Source: CAD feature listing. Evaluate the final solid. Frame: model axes, mm. Face numbers are marked on the shaded views. A direction names the side the tool comes from. Round coordinates to 2 decimals unless told otherwise and drop trailing zeros. Order: outer loops, then holes, each group sorted by start corner. A loop starts at its lowest first (then second) coordinate and runs counter-clockwise, first axis right, second up. Notation, with made-up numbers: (48, -7) -> (65, -7) arc R17 cw to (65, 11) -> close; hole circle Ø7 at (37, -23.75). An arc over 180 degrees is marked (long way). Write item = value, one per line. Start each with the question number.
(1) Cut plane B-B on y = 38. Return the cut outline in (x, z).
(2) Ray query, line 1 (Y direction, x = 43.5, z = 45.5); line 2 (Z direction, x = 41.5, y = -24); line 3 (Z direction, x = -2.5, y = -39). Return the intervals inside material, ascending.
(3) Cut plane A-A on x = -25.5. Return the cut outline in (y, z).
(4) Cut plane C-C on z = 36. Return the cut outline in (x, y), then the cut area to 3 significant figures.
(5) Contact query for flat-ended pins moving along their axis: pin 1 Ø6 at (x, y) = (-11, -40.5) entering from +Z; pin 2 Ø9 at (x, y) = (12, -28) entering from +Z; pin 3 Ø2.5 at (x, z) = (15, 53.5) entering from +Y. Output: stop coordinate, or through.
(6) Reachability of the marked faces 1, 2 and 3 from +Z, -Z, +X, -X, +Y, -Y: full face, straight path, thin tool, end or side. Return the list, or none.
from build123d import *

# Parameters (mm, degrees)
F0_W     = 100
F0_H     = 45
F1_DEPTH = 59
F0_H_2   = 11.5
F2_DEPTH = 50
F0_H_3   = 12.5
F3_DEPTH = 30.4


with BuildPart() as f1:
    # F0 (on Top) → F1 (new body)
    with BuildSketch(Plane.XY):
        Rectangle(F0_W, F0_H)
    extrude(amount=F1_DEPTH)

    # F0 (on Top) → F2 (join)
    with BuildSketch(Plane.XY):
        with Locations((0, 28.25)):
            Rectangle(F0_W, F0_H_2)
        with Locations((0, -28.25)):
            Rectangle(F0_W, F0_H_2)
    extrude(amount=F2_DEPTH)

    # F0 (on Top) → F3 (join)
    with BuildSketch(Plane.XY):
        with Locations((0, 40.25)):
            Rectangle(F0_W, F0_H_3)
        with Locations((0, -40.25)):
            Rectangle(F0_W, F0_H_3)
    extrude(amount=F3_DEPTH)


solid = f1.part
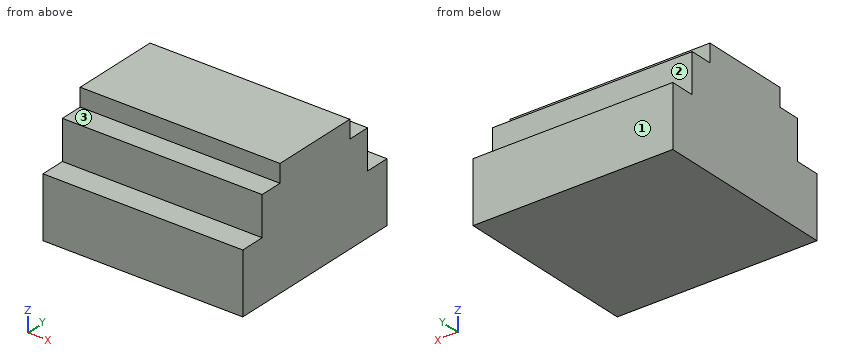
Evaluation:
q1.outline = (-50, 0) -> (50, 0) -> (50, 30.4) -> (-50, 30.4) -> close
q2.line_1 = -34 to 34
q2.line_2 = 0 to 50
q2.line_3 = 0 to 30.4
q3.outline = (-46.5, 0) -> (46.5, 0) -> (46.5, 30.4) -> (34, 30.4) -> (34, 50) -> (22.5, 50) -> (22.5, 59) -> (-22.5, 59) -> (-22.5, 50) -> (-34, 50) -> (-34, 30.4) -> (-46.5, 30.4) -> close
q4.outline = (-50, -34) -> (50, -34) -> (50, 34) -> (-50, 34) -> close
q4.area = 6,800 mm^2
q5.pin_1 = 30.4
q5.pin_2 = 50
q5.pin_3 = 22.5
q6.face_1 = +Z, -Z, +X, -X, +Y
q6.face_2 = +Z, +X, -X, +Y
q6.face_3 = +Z, +X, -X, -Y
